CAD build for the part. Positions are in the model's coordinates, mm. Face numbers are marked on the shaded views. A direction names the side the tool comes from. Give positions to 0.01 mm unless a question says otherwise; leave off trailing zeros. Order: outer loops, then holes, each group sorted by start corner. A loop starts at its lowest first (then second) coordinate and runs counter-clockwise, first axis right, second up.
from build123d import *

# Parameters (mm, degrees)
SKETCH_R        = 4.15
EXTRUDE_DEPTH   = 7
SKETCH001_R     = 1.55
POCKET_DEPTH    = 4
SKETCH002_R     = 2
POCKET001_DEPTH = 27.5798157383
POCKET002_DEPTH = 3.5
POCKET003_DEPTH = 2.25
POCKET004_DEPTH = 2.6


with BuildPart() as part:
    # Sketch → Extrude (new body)
    with BuildSketch(Plane.XY):
        with BuildLine():
            ThreePointArc((4.5, -13.6788157382), (0, 14.4), (-4.5, -13.6788157382))
            Line((-4.5, -13.6788157382), (-4.5, -17.1788157382))
            Line((-4.5, -17.1788157382), (4.5, -17.1788157382))
            Line((4.5, -17.1788157382), (4.5, -13.6788157382))
        make_face()
        Circle(SKETCH_R, mode=Mode.SUBTRACT)
        with BuildLine():
            ThreePointArc((-4.1103420039, 6.4519445605), (-7.65, 0), (-4.1103420039, -6.4519445605))
            ThreePointArc((-5.856565731, -9.1929667594), (-3.612942768, -8.6955675235), (-4.1103420039, -6.4519445605))
            ThreePointArc((-5.856565731, 9.1929667594), (-10.9, 0), (-5.856565731, -9.1929667594))
            ThreePointArc((-4.1103420039, 6.4519445605), (-3.612942768, 8.6955675235), (-5.856565731, 9.1929667594))
        make_face(mode=Mode.SUBTRACT)
        with BuildLine():
            ThreePointArc((4.1103420039, -6.4519445605), (7.65, 0), (4.1103420039, 6.4519445605))
            ThreePointArc((5.856565731, 9.1929667594), (3.612942768, 8.6955675235), (4.1103420039, 6.4519445605))
            ThreePointArc((5.856565731, -9.1929667594), (10.9, 0), (5.856565731, 9.1929667594))
            ThreePointArc((4.1103420039, -6.4519445605), (3.612942768, -8.6955675235), (5.856565731, -9.1929667594))
        make_face(mode=Mode.SUBTRACT)
    extrude(amount=EXTRUDE_DEPTH)

    # Sketch001 → Pocket (cut)
    with BuildSketch(Plane.XZ.offset(17.1788157382)):
        with Locations((0, 3.5)):
            Circle(SKETCH001_R)
    extrude(amount=-POCKET_DEPTH, mode=Mode.SUBTRACT)

    # Sketch002 → Pocket001 (cut, through all)
    with BuildSketch(Plane.XZ.offset(13.1788157382)):
        with Locations((0, 3.5)):
            Circle(SKETCH002_R)
    extrude(amount=-POCKET001_DEPTH, mode=Mode.SUBTRACT)

    # Sketch003 → Pocket002 (cut)
    with BuildSketch(Plane.XY.offset(7)):
        Polygon((1.55, -17.1788157382), (-1.55, -17.1788157382), (-1.55, -13.1788157382), (-3.125, -13.1788157382), (-3.125, -10.9288157382), (3.125, -10.9288157382), (3.125, -13.1788157382), (1.55, -13.1788157382), align=None)
    extrude(amount=-POCKET002_DEPTH, mode=Mode.SUBTRACT)

    # Sketch004 → Pocket003 (cut)
    with BuildSketch(Plane.XZ.offset(10.9288157382)):
        with BuildLine():
            Line((-3.125, 3.5), (3.125, 3.5))
            ThreePointArc((-3.125, 3.5), (0, 0.375), (3.125, 3.5))
        make_face()
    extrude(amount=POCKET003_DEPTH, mode=Mode.SUBTRACT)

    # Sketch005 → Pocket004 (cut)
    with BuildSketch(Plane.XY.offset(7)):
        with BuildLine():
            ThreePointArc((-3.4521499836, 5.4187900393), (-6.425, 0), (-3.4521499836, -5.4187900393))
            Line((-3.4521499836, -5.4187900393), (-2.064393013, -6.3028887726))
            Line((-2.064393013, -6.3028887726), (-2.1361664367, -7.9467709324))
            Line((-2.1361664367, -7.9467709324), (-2.2079398605, -9.5906530922))
            Line((-2.2079398605, -9.5906530922), (-3.6674703033, -10.3504365259))
            Line((-3.6674703033, -10.3504365259), (-5.1270007461, -11.1102199597))
            Line((-5.1270007461, -11.1102199597), (-6.5147577512, -10.2261212805))
            ThreePointArc((-6.5147577512, 10.2261212805), (-12.125, 0), (-6.5147577512, -10.2261212805))
            Line((-6.5147577512, 10.2261212805), (-5.1270007739, 11.1102200297))
            Line((-5.1270007739, 11.1102200297), (-3.6674703412, 10.3504365457))
            Line((-3.6674703412, 10.3504365457), (-2.2079399085, 9.5906530616))
            Line((-2.2079399085, 9.5906530616), (-2.1361664349, 7.9467708897))
            Line((-2.1361664349, 7.9467708897), (-2.0643929612, 6.3028887178))
            Line((-2.0643929612, 6.3028887178), (-3.4521499836, 5.4187900393))
        make_face()
        with BuildLine():
            ThreePointArc((3.4521499836, -5.4187900393), (6.425, 0), (3.4521499836, 5.4187900393))
            Line((3.4521499836, 5.4187900393), (2.0643912497, 6.3028869075))
            Line((2.0643912497, 6.3028869075), (2.1361663732, 7.9467694786))
            Line((2.1361663732, 7.9467694786), (2.2079414968, 9.5906520497))
            Line((2.2079414968, 9.5906520497), (3.667471594, 10.3504371978))
            Line((3.667471594, 10.3504371978), (5.1270016912, 11.110222346))
            Line((5.1270016912, 11.110222346), (6.5147577512, 10.2261212805))
            ThreePointArc((6.5147577512, -10.2261212805), (12.125, 0), (6.5147577512, 10.2261212805))
            Line((5.1270027116, -11.1102249223), (6.5147577512, -10.2261212805))
            Line((3.6674729876, -10.3504379233), (5.1270027116, -11.1102249223))
            Line((2.2079432635, -9.5906509242), (3.6674729876, -10.3504379233))
            Line((2.1361663047, -7.9467679091), (2.2079432635, -9.5906509242))
            Line((2.0643893459, -6.3028848939), (2.1361663047, -7.9467679091))
            Line((3.4521499836, -5.4187900393), (2.0643893459, -6.3028848939))
        make_face()
    extrude(amount=-POCKET004_DEPTH, mode=Mode.SUBTRACT)


solid = part.part
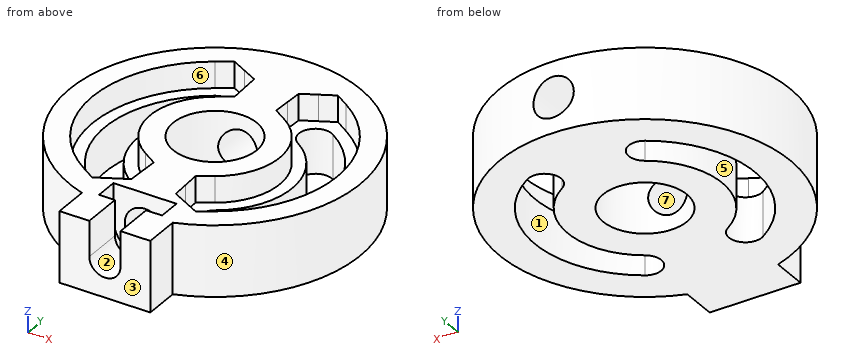
1. Saw through at A-A on z = 4. State how many separate pieces and enclosed holes the cut face has, plus the area to 3 significant figures.
2. Pin check, flat tips, straight feed: P1, Ø2.5, axis at y = -12, z = 4.5, coming from the +X side; P2, Ø2.5, axis at x = 0, z = 3.5, coming from the -Y side; P3, Ø3, axis at x = -0.5, y = -6.5, coming from the -Z side; P4, Ø1.8, axis at y = -15, z = 4.5, coming from the +X side. Stop position of each tip, or through.
3. Wall check: line 1 (Z direction, x = 0, y = 6.5); line 2 (X direction, y = -7, z = 3.5); line 3 (X direction, y = 7.5, z = 5). Give the ranges that are in metal, low to high.
4. Saw through at B-B on y = -8.5. Give the cut face in (x, z), plus the area to 3 significant figures.
5. Mould opens along X. For the marked faces 1, 2, 3 and 4 say: released by +X, released by -X, zero draft, split by the parting line, or undercut.
6. Saw through at D-D on y = 0. Give the cut face in (x, z) (3 decimals).
7. Saw through at C-C on x = 0. Give the cut face in (y, z) (3 decimals).
8. 3-axis set-ups, long thin cutter, end or side, ignore diameter. For the marked faces 5, 6 and 7: which of +Z, -Z, +X, -X, +Y, -Y reach the whole face in a straight line?
Reported:
1. separate pieces: 2
1. enclosed holes: 2
1. area: 393 mm2
2. P1: stops at x = 9.58
2. P2: passes through
2. P3: stops at z = 0
2. P4: stops at x = 4.5
3. line 1: z = 0 to 1.5, 5.5 to 7
3. line 2: x = -12.58 to -8.36, -3.58 to -2, 2 to 3.58, 8.36 to 12.58
3. line 3: x = -12.29 to -9.53, -2.12 to -1.32, 1.32 to 2.12, 9.53 to 12.29
4. outline: (-11.62, 0) - (-6.82, 0) - (-6.82, 4.4) - (-8.65, 4.4) - (-8.65, 7) - (-11.62, 7) - close; (-3.51, 0) - (3.51, 0) - (3.51, 4.4) - (2.16, 4.4) - (2.16, 7) - (-2.16, 7) - (-2.16, 4.4) - (-3.51, 4.4) - close; (6.82, 0) - (11.62, 0) - (11.62, 7) - (8.65, 7) - (8.65, 4.4) - (6.82, 4.4) - close; hole circle Ø4 at (0, 3.5)
4. area: 87.2 mm2
5. face 1: undercut
5. face 2: undercut
5. face 3: zero draft
5. face 4: split by the parting line
6. outline: (-14.4, 0) - (-10.9, 0) - (-10.9, 4.4) - (-12.125, 4.4) - (-12.125, 7) - (-14.4, 7) - close; (-7.65, 0) - (-4.15, 0) - (-4.15, 7) - (-6.425, 7) - (-6.425, 4.4) - (-7.65, 4.4) - close; (4.15, 0) - (7.65, 0) - (7.65, 4.4) - (6.425, 4.4) - (6.425, 7) - (4.15, 7) - close; (10.9, 0) - (14.4, 0) - (14.4, 7) - (12.125, 7) - (12.125, 4.4) - (10.9, 4.4) - close
7. outline: (-17.179, 0) - (-4.15, 0) - (-4.15, 1.5) - (-10.929, 1.5) - (-10.929, 0.375) - (-13.179, 0.375) - (-13.179, 1.95) - (-17.179, 1.95) - close; (-10.929, 5.5) - (-4.15, 5.5) - (-4.15, 7) - (-10.929, 7) - close; (4.15, 0) - (14.4, 0) - (14.4, 1.5) - (4.15, 1.5) - close; (4.15, 5.5) - (14.4, 5.5) - (14.4, 7) - (4.15, 7) - close
8. face 5: +Z, -Z
8. face 6: +Z
8. face 7: +Y
